Autodesk Inventor part; units mm, degrees
ref_plane "Work Plane2" through (-5.2503, 8.15, -5.2503) normal (0, 1, 0) x (-0.7071, 0, 0.7071)
ref_plane "YZ Plane" through (0, 0, 0) normal (1, 0, 0) x (0, 1, 0)
ref_plane "XZ Plane" through (0, 0, 0) normal (0, 1, 0) x (-1, 0, 0)
sketch "Sketch1" plane through (0, 0, 0) normal (0, 1, 0) x (-1, 0, 0)
  line L0 (-80.6, -80.6) -> (80.6, -80.6)
  line L1 (80.6, -80.6) -> (80.6, 80.6)
  line L2 (80.6, 80.6) -> (-80.6, 80.6)
  line L3 (-80.6, 80.6) -> (-80.6, -80.6)
  line L4 (-80.6, -80.6) -> (80.6, 80.6) construction
  line L5 (80.6, -80.6) -> (-80.6, 80.6) construction
  point P0 (0, 0)
  dimension "d0" = 161.2
extrude "Extrusion1" add sketch "Sketch1" along normal blind 3
sketch "Sketch2" plane through (0, 3, 0) normal (0, 1, 0) x (1, 0, 0)
  line L0 (-80.6, 80.6) -> (-80.6, -80.6)
  line L1 (-80.6, -80.6) -> (80.6, -80.6)
  line L2 (80.6, -80.6) -> (80.6, 80.6)
  line L3 (80.6, 80.6) -> (-80.6, 80.6)
  line L4 (77.6, 77.6) -> (-77.6, 77.6)
  line L5 (-77.6, 77.6) -> (-77.6, -77.6)
  line L6 (-77.6, -77.6) -> (77.6, -77.6)
  line L7 (77.6, -77.6) -> (77.6, 77.6)
  line L8 (77.6, 77.6) -> (-77.6, -77.6) construction
  line L9 (-77.6, 77.6) -> (77.6, -77.6) construction
  point P0 (0, 0)
  dimension "d3" = 3
  dimension "d4" = 3
extrude "Extrusion2" add sketch "Sketch2" along normal blind 62
sketch "Sketch3" plane through (0, 3, 0) normal (0, 1, 0) x (1, 0, 0)
  circle A0 centre (0, 0) radius 14
  dimension "d7" = 28
extrude "Extrusion3" cut sketch "Sketch3" against normal blind 44.5
ref_plane "Work Plane1" through (0, 38, 0) normal (0, 1, 0) x (1, 0, 0)
sketch "Sketch4" plane through (0, 38, 0) normal (0, 1, 0) x (1, 0, 0)
  line L0 (-77.6, -40.6) -> (-77.6, -72.6)
  line L1 (-77.6, -72.6) -> (-72.6, -77.6) construction
  line L2 (-72.6, -77.6) -> (-40.6, -77.6)
  line L3 (-40.6, -77.6) -> (-35.6, -72.6) construction
  line L4 (-35.6, -72.6) -> (-35.6, -40.6)
  line L5 (-35.6, -40.6) -> (-40.6, -35.6)
  line L6 (-40.6, -35.6) -> (-72.6, -35.6)
  line L7 (-72.6, -35.6) -> (-77.6, -40.6) construction
  circle A0 centre (-72.1, -41.1) radius 1.5
  circle A1 centre (-72.1, -72.1) radius 1.5
  circle A2 centre (-41.1, -72.1) radius 1.5
  circle A3 centre (-41.1, -41.1) radius 1.5
  circle A4 centre (-56.6, -56.6) radius 11 construction
  line L8 (-38.1, -75.1) -> (-75.1, -38.1) construction
  arc A5 (-65.0853, -48.1147) -> (-48.1147, -65.0853) centre (-56.6, -56.6) ccw
  arc A6 (-48.1147, -65.0853) -> (-65.0853, -48.1147) centre (-56.6, -56.6) ccw construction
  line L9 (-65.0853, -48.1147) -> (-65.0853, -35.6)
  line L10 (-48.1147, -65.0853) -> (-35.6, -65.0853)
  line L11 (-77.6, -77.6) -> (-77.6, 77.6)
  line L12 (77.6, -77.6) -> (-77.6, -77.6)
  line L13 (-35.6, -72.6) -> (-35.6, -77.6)
  line L14 (-72.6, -35.6) -> (-77.6, -35.6)
  point P0 (0, 0)
  dimension "d11" = 24
extrude "Extrusion4" add sketch "Sketch4" along normal blind 4 contours L11 L14 L6 L9 A5 L10 L4 L13 L12 L2 L0
sketch "Sketch5" plane through (0, 3, 0) normal (0, 1, 0) x (1, 0, 0)
  circle A0 centre (0, 0) radius 14
  line L0 (77.6, 77.6) -> (-77.6, 77.6)
  line L1 (-77.6, 77.6) -> (-77.6, -77.6)
  line L2 (-77.6, -77.6) -> (77.6, -77.6)
  line L3 (77.6, -77.6) -> (77.6, 77.6)
  circle A1 centre (0, 0) radius 17
  dimension "d14" = 3
ref_plane "Work Plane2" through (-5.2503, 8.15, -5.2503) normal (0, 1, 0) x (-0.7071, 0, 0.7071)
extrude "Extrusion5" add sketch "Sketch5" along normal up to surface (5.15 mm away) contours A1
sketch "Sketch6" plane through (0, 8.15, 0) normal (0, 1, 0) x (1, 0, 0)
  circle A0 centre (0, 0) radius 17
  circle A1 centre (0, 0) radius 8
  point P0 (0, 0)
  dimension "d17" = 16
extrude "Extrusion6" add sketch "Sketch6" along normal blind 5
sketch "Sketch7" plane through (0, 13.15, 0) normal (0, 1, 0) x (1, 0, 0)
  circle A0 centre (0, 0) radius 17
  circle A1 centre (0, 0) radius 3
  point P0 (0, 0)
  dimension "d20" = 6
extrude "Extrusion7" add sketch "Sketch7" along normal blind 24
sketch "Sketch9" plane through (0, 37.15, 0) normal (0, 1, 0) x (1, 0, 0)
  circle A0 centre (0, 0) radius 8
  circle A1 centre (0, 0) radius 17
  point P0 (0, 0)
  dimension "d23" = 16
extrude "Extrusion8" add sketch "Sketch9" along normal blind 5
equation "\"d0\" = Lenght"
equation "\"d1\" = Gr"
equation "\"d3\" = Gr"
equation "\"d4\" = Gr"
equation "\"d14\" = Gr"
equation "\"d17\" = bearing"
equation "\"d23\" = bearing"
equation "\"Gr\" = 3"
equation "\"Lenght\" = 161.2"
equation "\"bearing\" = 16"
properties part number "Base"
For this review, take the finished solid that the model builds, in its own axes (mm). A direction names the side the tool comes from. Give positions to 0.01 mm unless a question says otherwise; leave off trailing zeros. Write each loop counter-clockwise with the first axis right and the second up, starting at its lowest first coordinate (ties: lowest second). Pieces come first, ordered by that corner, then holes.
Item 1: Wall thickness on probe 1 along X at (y, z) = (5, 0); probe 2 along Z at (x, y) = (0, 21): over which ranges is each line inside the solid? List them lowest first.
Item 2: Take a section at C-C (y = 61.5). Give the boundary of the cut face in (x, z), and give its area (3 significant figures).
Item 3: Insertion check: P1, Ø2.5, axis at x = -72.1, z = 41.1, coming from the +Y side; P2, Ø17, axis at x = 6, z = 7, coming from the +Y side; P3, Ø8, axis at x = 0.5, z = -1, coming from the +Y side. Each pin has a flat end and moves straight along its axis. Give the tip position at first contact, or say it passes through.
Item 4: Take a section at D-D (x = 71). Give the boundary of the cut face in (y, z), and give its area (3 significant figures).
Item 5: Take a section at A-A (y = 6). Give the boundary of the cut face in (x, z).
Item 6: Machinability: for faces 1 (the face through (-77.6, 34, -1)), 2 (the face through (-1.73, 10.62, -7.81)), 3 (the face through (-66, 42, 66)), 4 (the face through (-17, 0, 1)), which of the approach directions +Z, -Z, +X, -X, +Y, -Y give a long, thin tool a straight path to every point of the face, cutting with its end or side? Answer none if there is none.
Item 7: Take a section at B-B (x = 0). Give the boundary of the cut face in (y, z), and give its area (3 significant figures).
Item 8: The part is to be moulded in two halves that separate along X. For faces 5 (the face through (-1, 32, 80.6)), 6 (the face through (6, 8.15, 6)), 7 (the face through (80.6, 32, 1)), say which applies: +X half, -X half, draft (parallel to the pull), parting line (faces both ways), or undercut.
Established:
1. probe 1: x = -80.6 to -77.6, -17 to -14, 14 to 17, 77.6 to 80.6
1. probe 2: z = -80.6 to -77.6, -17 to -3, 3 to 17, 77.6 to 80.6
2. outline: (-80.6, -80.6) - (80.6, -80.6) - (80.6, 80.6) - (-80.6, 80.6) - close; hole (-77.6, -77.6) - (77.6, -77.6) - (77.6, 77.6) - (-77.6, 77.6) - close
2. area: 1,900 mm2
3. P1: stops at y = 3
3. P2: stops at y = 42.15
3. P3: stops at y = 37.15
4. outline: (0, -80.6) - (65, -80.6) - (65, -77.6) - (3, -77.6) - (3, 77.6) - (65, 77.6) - (65, 80.6) - (0, 80.6) - close
4. area: 856 mm2
5. outline: (-80.6, -80.6) - (80.6, -80.6) - (80.6, 80.6) - (-80.6, 80.6) - close; circle Ø34 at (0, 0); hole (-77.6, -77.6) - (77.6, -77.6) - (77.6, 77.6) - (-77.6, 77.6) - close; hole circle Ø28 at (0, 0)
6. face 1: none
6. face 2: -Y
6. face 3: +Y
6. face 4: +Z, -Z, +X, -X, -Y
7. outline: (0, -80.6) - (65, -80.6) - (65, -77.6) - (3, -77.6) - (3, -17) - (42.15, -17) - (42.15, -8) - (37.15, -8) - (37.15, -3) - (13.15, -3) - (13.15, -8) - (8.15, -8) - (8.15, -14) - (0, -14) - close; (0, 14) - (8.15, 14) - (8.15, 8) - (13.15, 8) - (13.15, 3) - (37.15, 3) - (37.15, 8) - (42.15, 8) - (42.15, 17) - (3, 17) - (3, 77.6) - (65, 77.6) - (65, 80.6) - (0, 80.6) - close
7. area: 1,650 mm2
8. face 5: draft
8. face 6: undercut
8. face 7: +X half
